Answer from the drawing. Dimensions are ordinates in mm from the lowest x, y and z of the part. A direction names the side the tool comes from. Coordinates: 2 decimals unless noted, no trailing zeros. Order: outer loops, then holes, each group sorted by start corner. A loop starts at its lowest first (then second) coordinate and runs counter-clockwise, first axis right, second up. Notation, with made-up numbers: (-36, 46.5) -> (7, 46.5) arc R23 ccw to (7, 83.5) -> close; hole circle Ø4 at (40, 1.25). An arc over 180 degrees is marked (long way). Answer as a JSON object with one key per item and string values. Group by question number.
1) A tool of negligible diameter and unlimited length cuts with its end or side. For the marked faces 1, 2 and 3, from which of +Z, -Z, +X, -X, +Y, -Y can it reach the whole face along a straight path? Write none if from no direction.
2) Given pin 1 (7.5 mm diameter, centred on x = 9, z = 73, fed in from -Y); pin 2 (6.5 mm diameter, centred on x = 7.5, y = 8.5, fed in from +Z); pin 3 (7.5 mm diameter, centred on x = 7, y = 10.5, fed in from -Z); pin 4 (8 mm diameter, centred on y = 11, z = 22, fed in from -X), each flat-ended and moving along its own axis, determine where each tip first touches the part or whether it passes through.
3) Section B-B on z = 4 is taken. Determine the outline of the cut face in (x, y), and give its area (3 significant figures).
4) Section D-D on y = 1.5 is taken. Determine the outline of the cut face in (x, z).
5) Consider L1, parallel to Z at x = 7.5, y = 19.15; L2, parallel to Y at x = 7.5, z = 51.25; L3, parallel to Y at x = 12, z = 33. Determine where each line is inside the solid, lowest interval first.
6) Section C-C on x = 1.5 is taken. Determine the outline of the cut face in (y, z), and give its area (3 significant figures).
7) Section A-A on y = 8.5 is taken. Determine the outline of the cut face in (x, z).
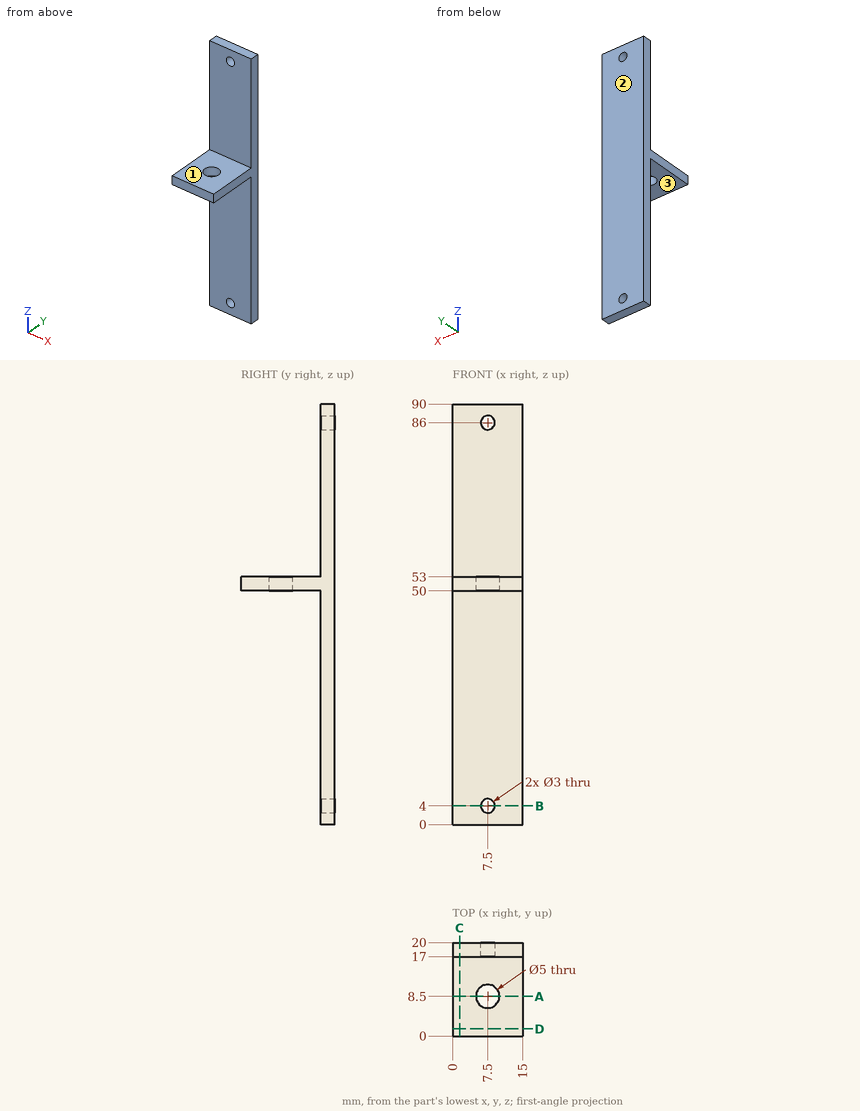
Worked answers:
{
 "1": {"face 1": "+Z, +X, -X, -Y", "face 2": "+Z, -Z, +X, -X, +Y", "face 3": "-Z, +X, -X, -Y"},
 "2": {"pin 1": "stops at y = 17", "pin 2": "stops at z = 53", "pin 3": "stops at z = 50", "pin 4": "passes through"},
 "3": {"outline": "(0, 17) -> (6, 17) -> (6, 20) -> (0, 20) -> close; (9, 17) -> (15, 17) -> (15, 20) -> (9, 20) -> close", "area": "36.0 mm²"},
 "4": {"outline": "(0, 50) -> (15, 50) -> (15, 53) -> (0, 53) -> close"},
 "5": {"L1": "z = 0 to 2.5, 5.5 to 84.5, 87.5 to 90", "L2": "y = 0 to 6, 11 to 20", "L3": "y = 17 to 20"},
 "6": {"outline": "(0, 50) -> (17, 50) -> (17, 0) -> (20, 0) -> (20, 90) -> (17, 90) -> (17, 53) -> (0, 53) -> close", "area": "321 mm²"},
 "7": {"outline": "(0, 50) -> (5, 50) -> (5, 53) -> (0, 53) -> close; (10, 50) -> (15, 50) -> (15, 53) -> (10, 53) -> close"}
}
